from build123d import *

# Parameters (mm, degrees)
F0_R     = 32.5
F1_DEPTH = 40
F2_R     = 22.5
F3_DEPTH = 40
F4_W     = 15
F4_H     = 40
F5_DEPTH = 32.5


with BuildPart() as f1:
    # F0 (on Top) → F1 (new body)
    with BuildSketch(Plane.XY):
        Circle(F0_R)
    extrude(amount=F1_DEPTH)

    # F2 (on face) → F3 (join)
    with BuildSketch(Plane.XY.offset(40)):
        Circle(F2_R)
    extrude(amount=F3_DEPTH)

    # F4 (on Right) → F5 (cut, symmetric)
    with BuildSketch(Plane.YZ):
        with Locations((0, 45)):
            Rectangle(F4_W, F4_H)
    extrude(amount=F5_DEPTH, both=True, mode=Mode.SUBTRACT)


solid = f1.part
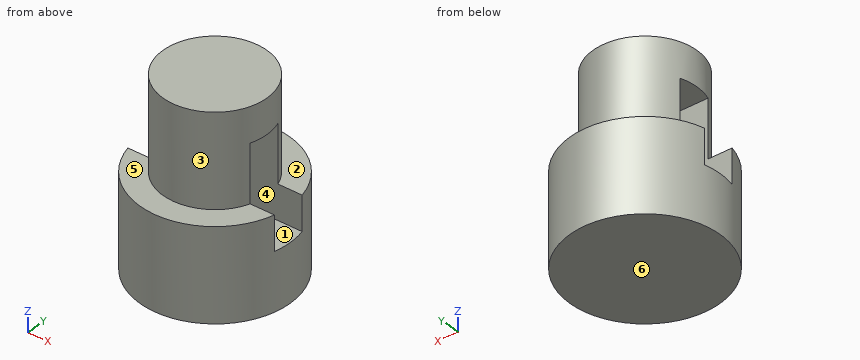
Geometry: final body of the model. Coordinates: model frame, mm. Face numbers are marked on the shaded views. A direction names the side the tool comes from. Give positions to 0.01 mm unless a question says otherwise; leave off trailing zeros. Loops run counter-clockwise (first coordinate to the right, second up) from the corner with the lowest first, then second, coordinate; pieces in that order, holes last. Notation, with made-up numbers: (-25.5, 23.5) - (1.5, 23.5) arc R18 cw to (1.5, 29.5) - close; hole circle Ø9 at (-16.5, -14). An arc over 180 degrees is marked (long way). One line per question, with ' | ' between items. Start each with the question number.
(1) Ray query, line 1 (Z direction, x = -17, y = 1); line 2 (Y direction, x = -1, z = 30.5); line 3 (Y direction, x = -0.5, z = 43.5). Return the intervals inside material, ascending. Write a range as from..to.
(2) Section query B-B on x = 0. Return loops of the section in (y, z), then the cut area to 3 significant figures.
(3) Section query D-D on x = 28. Return loops of the section in (y, z).
(4) Section query C-C on z = 31. Return loops of the section in (x, y).
(5) Contact query for flat-ended pins moving along their axis: pin 1 (3 mm diameter, centred on y = -1.5, z = 65, fed in from +X); pin 2 (1.5 mm diameter, centred on x = -7.5, z = 54, fed in from +Y); pin 3 (4 mm diameter, centred on y = -18, z = 31, fed in from -X). Output: stop coordinate, or through.
(6) Section query A-A on y = 0. Return loops of the section in (x, z), then the cut area to 3 significant figures.
(7) Pull-direction query (Z, two-part tool) for the marked faces 4, 5 and 6; classes: released by +Z, released by -Z, zero draft, split by the parting line, or undercut.
(8) Reachability of the marked faces 1, 2 and 3 from +Z, -Z, +X, -X, +Y, -Y: full face, straight path, thin tool, end or side. Return the list, or none.
The answers:
1) line 1: 0..25, 65..80 | line 2: -32.48..-7.5, 7.5..32.48 | line 3: -22.49..-7.5, 7.5..22.49
2) outline: (-32.5, 0) - (32.5, 0) - (32.5, 40) - (22.5, 40) - (22.5, 80) - (-22.5, 80) - (-22.5, 40) - (-32.5, 40) - close; hole (-7.5, 25) - (7.5, 25) - (7.5, 65) - (-7.5, 65) - close | area: 3,800 mm2
3) outline: (-16.5, 0) - (16.5, 0) - (16.5, 40) - (7.5, 40) - (7.5, 25) - (-7.5, 25) - (-7.5, 40) - (-16.5, 40) - close
4) outline: (-31.62, -7.5) arc R32.5 ccw to (31.62, -7.5) - close; (-31.62, 7.5) - (31.62, 7.5) arc R32.5 ccw to start
5) pin 1: x = 22.5 | pin 2: y = 21.46 | pin 3: x = -28.29
6) outline: (-32.5, 0) - (32.5, 0) - (32.5, 25) - (-32.5, 25) - close; (-22.5, 65) - (22.5, 65) - (22.5, 80) - (-22.5, 80) - close | area: 2,300 mm2
7) face 4: undercut | face 5: released by +Z | face 6: released by -Z
8) face 1: +X, -X | face 2: +Z, +Y | face 3: +Z
